Geometry: final body of the model. Coordinates: model frame, mm. Face numbers are marked on the shaded views. Coordinates: 2 decimals unless noted, no trailing zeros. Loops run counter-clockwise (first coordinate to the right, second up) from the corner with the lowest first, then second, coordinate; pieces in that order, holes last. Notation, with made-up numbers: M 8.5,-16 L 42.5,-16 A21 cw 42.5,3 Z; hole C 9,-23 d9. An arc over 180 degrees is marked long. Write each question's results on one line, items separated by ' | '. Start each with the question number.
from build123d import *

# Parameters (mm, degrees)
F1_DEPTH       = 420
F2_SIZE        = 3
F4_D           = 9
F4_CBORE_D     = 14
F4_CBORE_DEPTH = 10


with BuildPart() as f1:
    # F0 (on Front) → F1 (new body)
    with BuildSketch(Plane.XZ):
        Polygon((0, 2.400041), (30, 0), (40, 0), (40, 33), (35, 33), (35, 28), (5, 28), (5, 33), (0, 33), align=None)
    extrude(amount=F1_DEPTH)

    # F2
    f2_edges = [f1.edges().sort_by_distance(p)[0] for p in [
        (5, -210, 33),
        (35, -210, 33),
    ]]
    chamfer(f2_edges, length=F2_SIZE)

    # F4 (through all)
    with Locations(Plane.XY.offset(28)):
        with Locations((20, -390), (20, -270), (20, -150), (20, -30)):
            CounterBoreHole(F4_D / 2, F4_CBORE_D / 2, F4_CBORE_DEPTH)


solid = f1.part
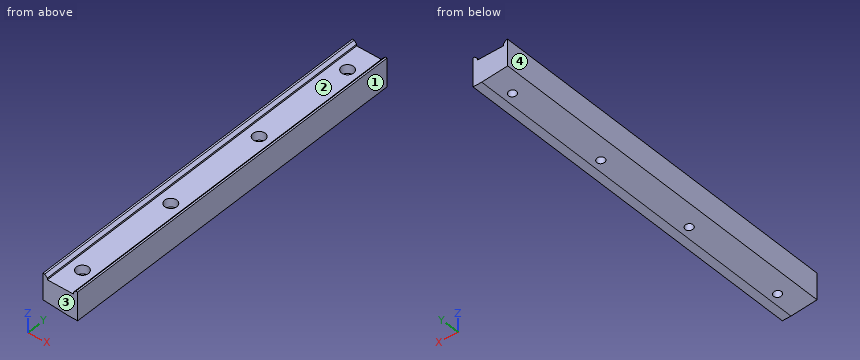
Item 1: Contact query for flat-ended pins moving along their axis: P1, Ø4, axis at x = 13, z = 5.5, coming from the +Y side; P2, Ø24, axis at x = 17.5, y = -105.5, coming from the +Z side; P3, Ø4, axis at x = 21, y = -29.5, coming from the +Z side; P4, Ø14.5, axis at x = 20, y = -150, coming from the -Z side. Output: stop coordinate, or through.
Item 2: Section B-B, the plane z = 24.5. Return loops of the section in (x, y), plus the area to 3 significant figures.
Item 3: Section D-D, the plane x = 21. Count the separate pieces of the cut face and the enclosed holes in it, plus the area to 3 significant figures.
Item 4: Ray query, L1, parallel to Y at x = 20, z = 25.75; L2, parallel to Y at x = 20, z = 9; L3, parallel to X at y = -270, z = 21.25. Return the intervals inside material, ascending. Write a range as [from, to].
Item 5: Section C-C, the plane y = -75.5. Return loops of the section in (x, z), plus the area to 4 significant figures.
Item 6: Section A-A, the plane y = -390. Return loops of the section in (x, z).
Item 7: Pull-direction query (X, two-part tool) for the marked faces 1, 2, 3 and 4; classes: released by +X, released by -X, zero draft, split by the parting line, or undercut.
Solutions:
1) P1: stops at y = 0 | P2: stops at z = 28 | P3: passes through | P4: stops at z = 0.22
2) outline: M 0,-420 L 40,-420 L 40,0 L 0,0 Z; hole C 20,-390 d14; hole C 20,-270 d14; hole C 20,-150 d14; hole C 20,-30 d14 | area: 16,200 mm²
3) separate pieces: 5 | enclosed holes: 0 | area: 10,300 mm²
4) L1: y = [-420, -397], [-383, -277], [-263, -157], [-143, -37], [-23, 0] | L2: y = [-420, -394.5], [-385.5, -274.5], [-265.5, -154.5], [-145.5, -34.5], [-25.5, 0] | L3: x = [0, 13], [27, 40]
5) outline: M 0,2.4 L 30,0 L 40,0 L 40,33 L 38,33 L 35,30 L 35,28 L 5,28 L 5,30 L 2,33 L 0,33 Z | area: 1,125 mm²
6) outline: M 0,2.4 L 15.5,1.16 L 15.5,18 L 13,18 L 13,28 L 5,28 L 5,30 L 2,33 L 0,33 Z; M 24.5,0.44 L 30,0 L 40,0 L 40,33 L 38,33 L 35,30 L 35,28 L 27,28 L 27,18 L 24.5,18 Z
7) face 1: released by +X | face 2: undercut | face 3: zero draft | face 4: released by -X
